Design review of the part built by this model. Coordinates are the model's own, in mm. A direction names the side the tool comes from. Coordinates: 2 decimals unless noted, no trailing zeros. Order: outer loops, then holes, each group sorted by start corner. A loop starts at its lowest first (then second) coordinate and runs counter-clockwise, first axis right, second up. Notation, with made-up numbers: (63.5, -9.5) -> (116.5, -9.5) arc R17 cw to (116.5, 11.5) -> close; hole circle Ø1 at (68.5, 25). An arc over 180 degrees is marked (long way). Write item = value, one per line.
Autodesk Inventor part; units mm, degrees
ref_plane "YZ Plane" through (0, 0, 0) normal (1, 0, 0) x (0, 1, 0)
ref_plane "XZ Plane" through (0, 0, 0) normal (0, 1, 0) x (-1, 0, 0)
ref_plane "XY Plane" through (0, 0, 0) normal (0, 0, 1) x (1, 0, 0)
sketch "Sketch1" plane through (0, 0, 0) normal (0, 0, 1) x (1, 0, 0)
  line L0 (-15, 7.5) -> (15, 7.5)
  line L1 (15, 7.5) -> (15, -7.5)
  line L2 (15, -7.5) -> (-15, -7.5)
  line L3 (-15, -7.5) -> (-15, 7.5)
  point P0 (0, 0)
  point P1 (-15, 0)
  point P2 (0, 7.5)
  dimension "d0" = 30
  dimension "d1" = 15
extrude "Extrusion1" add sketch "Sketch1" along normal blind 12.7
sketch "Sketch3" plane through (0, 0, 12.7) normal (0, 0, 1) x (1, 0, 0)
  line L0 (-15, 7.5) -> (15, 7.5)
  line L1 (15, -7.5) -> (-15, -7.5)
  line L2 (-6.477, 7.5) -> (6.477, 7.5)
  line L3 (6.477, 7.5) -> (6.477, -7.5)
  line L4 (6.477, -7.5) -> (-6.477, -7.5)
  line L5 (-6.477, -7.5) -> (-6.477, 7.5)
  point P0 (0, 0)
  point P1 (0, 7.5)
  dimension "d13" = 12.954
extrude "Extrusion2" cut sketch "Sketch3" against normal blind 9.525
sketch "Sketch4" plane through (0, 0, 0) normal (0, 0, -1) x (-1, 0, 0)
  point P0 (0, 0)
  point P1 (0, 0)
hole "Hole2" at (0, 0, 0) direction (0, 0, 1) diameter 4.9784 end through all
sketch "Sketch5" plane through (0, 0, 12.7) normal (0, 0, 1) x (1, 0, 0)
  point P0 (0, 0)
  point P1 (-11, 0)
  point P2 (11, 0)
  dimension "d23" = 11
  dimension "d24" = 11
hole "Hole3" at (-11, 0, 12.7) at (11, 0, 12.7) direction (0, 0, -1) diameter 3.4544 end through all counterbore diameter 6.5024 counterbore depth 6.35
chamfer "Chamfer1" distance 0.635 angle 45 2 edges at (6.477, 0, 12.7) (-6.477, 0, 12.7)
fillet "Fillet1" radius 3.175 4 edges at (15, 7.5, 6.35) (-15, 7.5, 6.35) (-15, -7.5, 6.35) (15, -7.5, 6.35)
properties part number "J002866" material "ALUMINUM, 6061-T651"
(1) We need section A-A (x = 0). Write out the cut boundary in (y, z) (3 decimals), and give its area (3 significant figures).
Report:
outline = (-7.5, 0) -> (-2.489, 0) -> (-2.489, 3.175) -> (-7.5, 3.175) -> close; (2.489, 0) -> (7.5, 0) -> (7.5, 3.175) -> (2.489, 3.175) -> close
area = 31.8 mm²
(2) We need section D-D (z = 2.25). Write out the cut boundary in (x, y) (3 decimals).
Report:
outline = (-15, -4.325) arc R3.175 ccw to (-11.825, -7.5) -> (11.825, -7.5) arc R3.175 ccw to (15, -4.325) -> (15, 4.325) arc R3.175 ccw to (11.825, 7.5) -> (-11.825, 7.5) arc R3.175 ccw to (-15, 4.325) -> close; hole circle Ø3.454 at (-11, 0); hole circle Ø4.978 at (0, 0); hole circle Ø3.454 at (11, 0)
(3) We need section C-C (y = 0). Give the number of separate pieces and of enclosed holes in the cut face, and give its area (3 significant figures).
Report:
separate_pieces = 4
enclosed_holes = 0
area = 115 mm²
(4) We need section B-B (z = 10.25). Write out the cut boundary in (x, y) (3 decimals), and give its area (3 significant figures).
Report:
outline = (-15, -4.325) arc R3.175 ccw to (-11.825, -7.5) -> (-6.477, -7.5) -> (-6.477, 7.5) -> (-11.825, 7.5) arc R3.175 ccw to (-15, 4.325) -> close; (6.477, -7.5) -> (11.825, -7.5) arc R3.175 ccw to (15, -4.325) -> (15, 4.325) arc R3.175 ccw to (11.825, 7.5) -> (6.477, 7.5) -> close; hole circle Ø6.502 at (-11, 0); hole circle Ø6.502 at (11, 0)
area = 181 mm²
(5) For faces 4 (the flat face through (-3, 0, 3.175)), 5 (the flat face through (-15, 0, 6)), 6 (the cylindrical face through (12.98, 2.58, 9.48)), list the 3-axis set-ups (+Z, -Z, +X, -X, +Y, -Y) from which the entire face can be reached by the end or side of a thin tool; tool diameter is ignored.
Report:
face_4 = +Z, +Y, -Y
face_5 = +Z, -Z, -X, +Y, -Y
face_6 = +Z
(6) For L1, parallel to X at y = 0, z = 9.75; L2, parallel to X at y = 0, z = 0.95; L3, parallel to X at y = 4, z = 7, list the stretches that pass through material, from the lowest coordinate up.
Report:
L1 = -15 to -14.25, -7.75 to -6.48, 6.48 to 7.75, 14.25 to 15
L2 = -15 to -12.73, -9.27 to -2.49, 2.49 to 9.27, 12.73 to 15
L3 = -15 to -6.48, 6.48 to 15
(7) The part is to be moulded in two halves that separate along X. For faces 1 (the cylindrical face through (-14.09, -6.55, 6.44)), 2 (the flat face through (15, 0, 6)), 3 (the cylindrical face through (-7.826, 0.705, 9.481)), say which applies: released by +X, released by -X, zero draft, split by the parting line, or undercut.
Report:
face_1 = released by -X
face_2 = released by +X
face_3 = undercut
(8) Insertion check: pin 1 (2 mm diameter, centred on x = 11, y = 0, fed in from -Z); pin 2 (5 mm diameter, centred on x = 10.5, y = -1.5, fed in from +Z); pin 3 (4 mm diameter, centred on x = 2.5, y = 0.5, fed in from +Z) (3 decimals); pin 4 (5 mm diameter, centred on x = -11, y = 0, fed in from +Z). Each pin has a flat end and moves straight along its axis. Give the tip position at first contact, or say it passes through.
Report:
pin_1 = through
pin_2 = 12.7
pin_3 = 3.175
pin_4 = 6.35
